Source: CAD feature listing. Evaluate the final solid. Frame: model axes, mm. Give positions to 0.01 mm unless a question says otherwise; leave off trailing zeros. Order: outer loops, then holes, each group sorted by start corner. A loop starts at its lowest first (then second) coordinate and runs counter-clockwise, first axis right, second up.
from build123d import *

# Parameters (mm, degrees)
BOSS_EXTRUDE1_DEPTH = 3.175
FILLET2_R           = 50.8
SKETCH2_W           = 127
SKETCH2_H           = 38.1
CUT_EXTRUDE1_DEPTH  = 4.175
FILLET3_R           = 6.35


with BuildPart() as part:
    # Sketch1 → Boss-Extrude1 (new body)
    with BuildSketch(Plane.XY):
        Polygon((-304.8, 1009.65), (304.8, 1009.65), (698.5, 596.9), (698.5, 0), (-698.5, 0), (-698.5, 596.9), align=None)
    extrude(amount=BOSS_EXTRUDE1_DEPTH)

    # Fillet2
    fillet2_edges = [part.edges().sort_by_distance(p)[0] for p in [
        (698.5, 596.9, 1.5875),
        (-698.5, 596.9, 1.5875),
        (-304.8, 1009.65, 1.5875),
        (304.8, 1009.65, 1.5875),
    ]]
    fillet(fillet2_edges, radius=FILLET2_R)

    # Sketch2 → Cut-Extrude1 (cut, through all)
    with BuildSketch(Plane(origin=(0, 0, 0), x_dir=(-1, 0, 0), z_dir=(0, 0, -1))):
        with Locations((374.65, 19.05)):
            Rectangle(SKETCH2_W, SKETCH2_H)
        with Locations((-374.65, 19.05)):
            Rectangle(SKETCH2_W, SKETCH2_H)
    extrude(amount=-CUT_EXTRUDE1_DEPTH, mode=Mode.SUBTRACT)

    # Fillet3
    fillet3_edges = [part.edges().sort_by_distance(p)[0] for p in [
        (-311.15, 0, 1.5875),
        (-311.15, 38.1, 1.5875),
        (-438.15, 38.1, 1.5875),
        (-438.15, 0, 1.5875),
        (311.15, 0, 1.5875),
        (438.15, 0, 1.5875),
        (438.15, 38.1, 1.5875),
        (311.15, 38.1, 1.5875),
    ]]
    fillet(fillet3_edges, radius=FILLET3_R)


solid = part.part
1) First-contact query: pin 1 Ø1.5 at (y, z) = (659, 2.5) entering from -X. Flat tip, straight axial feed; report the tip coordinate or a pass-through.
Checks:
pin 1: stops at x = -639.98
2) Ray query, L1, parallel to X at y = 810.5, z = 2.8; L2, parallel to X at y = 784, z = 2.4; L3, parallel to Y at x = -358, z = 1.15. Return the intervals inside material, ascending.
Checks:
L1: x = -494.76 to 494.76
L2: x = -520.04 to 520.04
L3: y = 38.1 to 953.88
3) Section query C-C on x = 518. Output: boundary loops of the cut face in (y, z) (3 decimals).
Checks:
outline: (0, 0) - (786.134, 0) - (786.134, 3.175) - (0, 3.175) - close
4) Section query B-B on y = 740.5. Output: boundary loops of the cut face in (x, z) (3 decimals).
Checks:
outline: (-561.528, 0) - (561.528, 0) - (561.528, 3.175) - (-561.528, 3.175) - close
5) Section query A-A on z = 2.1. Output: boundary loops of the cut face in (x, y), and give its area (3 significant figures).
Checks:
outline: (-698.5, 0) - (-444.5, 0) arc R6.35 ccw to (-438.15, 6.35) - (-438.15, 31.75) arc R6.35 cw to (-431.8, 38.1) - (-317.5, 38.1) arc R6.35 cw to (-311.15, 31.75) - (-311.15, 6.35) arc R6.35 ccw to (-304.8, 0) - (304.8, 0) arc R6.35 ccw to (311.15, 6.35) - (311.15, 31.75) arc R6.35 cw to (317.5, 38.1) - (431.8, 38.1) arc R6.35 cw to (438.15, 31.75) - (438.15, 6.35) arc R6.35 ccw to (444.5, 0) - (698.5, 0) - (698.5, 576.56) arc R50.8 ccw to (684.46, 611.62) - (319.81, 993.91) arc R50.8 ccw to (283.05, 1009.65) - (-283.05, 1009.65) arc R50.8 ccw to (-319.81, 993.91) - (-684.46, 611.62) arc R50.8 ccw to (-698.5, 576.56) - close
area: 1,240,000 mm2
